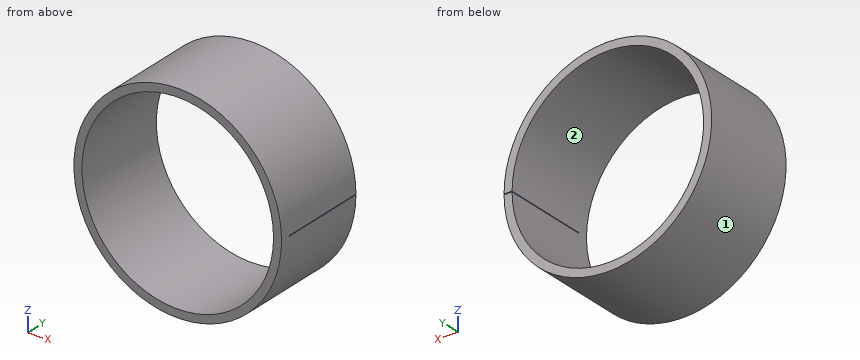
```python
from build123d import *

# Parameters (mm, degrees)
F0_R     = 8.5625
F0_R_2   = 7.9
F1_DEPTH = 8.05
F3_DEPTH = 25
F5_SCALE = 25.4


with BuildPart() as f1:
    # F0 (on Front) → F1 (new body)
    with BuildSketch(Plane.XZ):
        Circle(F0_R)
        Circle(F0_R_2, mode=Mode.SUBTRACT)
    extrude(amount=F1_DEPTH)

    # F2 (on Right) → F3 (cut)
    with BuildSketch(Plane.YZ):
        with BuildLine():
            Line((0.064567852, 0.03), (0, 0.03))
            Line((0, 0.03), (-7.0868510798, 0.03))
            ThreePointArc((-7.0868510798, 0.03), (-7.204668453, 0), (-7.0868510798, -0.03))
            Line((-7.0868510798, -0.03), (0, -0.03))
            Line((0, -0.03), (0.064567852, -0.0370406015))
            Line((0.064567852, -0.0370406015), (0.064567852, 0.03))
        make_face()
    extrude(amount=F3_DEPTH, mode=Mode.SUBTRACT)


with BuildPart() as f1_1:
    # F5: moved
    add(f1.part.scale(F5_SCALE).moved(Location((5.408359057, 0, 0))))


solid = f1_1.part
```
Geometry check sheet. Reference: the model listing, model coordinates, mm. Face numbers are marked on the shaded views. Round coordinates to 2 decimals unless told otherwise and drop trailing zeros. Order: outer loops, then holes, each group sorted by start corner. A loop starts at its lowest first (then second) coordinate and runs counter-clockwise, first axis right, second up. Notation, with made-up numbers: (-10.5, 36) - (30.5, 36) arc R26 ccw to (30.5, 69) - close; hole circle Ø1 at (86.5, 68). An arc over 180 degrees is marked (long way). Use a Markdown table: item, result. Add a question column.
(1) Release check for a two-part mould opening along Z. For the marked faces 1 and 2 record: pulls with the +Z half, pulls with the -Z half, needs draft (parallel to the pull), parting line crosses it, or undercut.
(2) Sectioned sample at C-C, the plane y = -41.5. Enter the section's corners in (x, z) (1 decimal), and give its area (3 significant figures).
(3) Sectioned sample at A-A, the plane x = -41.5. Enter the section's corners in (y, z), and give its area (3 significant figures).
(4) Sectioned sample at B-B, the plane z = -95. Enter the section's corners in (x, y).
(5) Depth check by flat-ended pin: pin 1 (8 mm diameter, centred on y = -181.5, z = 108.5, fed in from +X); pin 2 (5 mm diameter, centred on x = -116.5, y = -178, fed in from +Z); pin 3 (4 mm diameter, centred on x = 74, y = -115, fed in from -Z); pin 4 (1 mm diameter, centred on x = 142.5, z = 171, fed in from -Y). Enter the tip coordinate at first touch or a pass-through.
(6) Material ranges on line 1 along Z through (x, y) = (1.5, -20); line 2 along Z through (x, y) = (156.5, -156); line 3 along X through (y, z) = (-32.5, -158), recorded low to high. Write a range as [from, to].
Answers below:
| question | item | result |
|---|---|---|
| 1 | face 1 | parting line crosses it |
| 1 | face 2 | undercut |
| 2 | outline | (206.1, -0.8) arc R200.7 cw (long way) to (206.1, 0.8) - (222.9, 0.8) arc R217.5 ccw (long way) to (222.9, -0.8) - close |
| 2 | area | 22,100 mm² |
| 3 | outline | (-204.47, -212.37) - (0, -212.37) - (0, -195.1) - (-204.47, -195.1) - close; (-204.47, 195.1) - (0, 195.1) - (0, 212.37) - (-204.47, 212.37) - close |
| 3 | area | 7,060 mm² |
| 4 | outline | (-190.23, -204.47) - (-171.34, -204.47) - (-171.34, 0) - (-190.23, 0) - close; (182.16, -204.47) - (201.05, -204.47) - (201.05, 0) - (182.16, 0) - close |
| 5 | pin 1 | x = 196.15 |
| 5 | pin 2 | z = 181.78 |
| 5 | pin 3 | z = -207.04 |
| 5 | pin 4 | through |
| 6 | line 1 | [-217.45, -200.62], [200.62, 217.45] |
| 6 | line 2 | [-156.44, -132.04], [132.04, 156.44] |
| 6 | line 3 | [-144.05, -118.29], [129.1, 154.86] |
